Read the model definition and answer for the solid it produces. Units are mm, in the model's axes. A direction names the side the tool comes from. Coordinates: 2 decimals unless noted, no trailing zeros. Order: outer loops, then holes, each group sorted by start corner. A loop starts at its lowest first (then second) coordinate and runs counter-clockwise, first axis right, second up.
```python
from build123d import *

# Parameters (mm, degrees)
F1_W     = 21
F1_H     = 35
F2_DEPTH = 23
F3_W     = 19
F3_H     = 33
F4_DEPTH = 22
F5_W     = 7
F5_H     = 14.7
F6_DEPTH = 25
F8_D     = 4
F8_DEPTH = 6
F8_TIP   = 1.2017212381


with BuildPart() as f2:
    # F1 (on Front) → F2 (new body)
    with BuildSketch(Plane.XZ):
        Rectangle(F1_W, F1_H)
    extrude(amount=-F2_DEPTH)

    # F3 (on face) → F4 (cut)
    with BuildSketch(Plane(origin=(0, 23, 0), x_dir=(-1, 0, 0), z_dir=(0, 1, 0))):
        Rectangle(F3_W, F3_H)
    extrude(amount=-F4_DEPTH, mode=Mode.SUBTRACT)

    # F5 (on Front) → F6 (cut)
    with BuildSketch(Plane.XZ):
        Rectangle(F5_W, F5_H)
    extrude(amount=-F6_DEPTH, mode=Mode.SUBTRACT)

    # F8
    with Locations(Plane.XZ):
        with Locations((0, 14.35), (-6, 0), (6, 0), (0, -14.35)):
            Hole(F8_D / 2, depth=F8_DEPTH)
            with Locations((0, 0, -(F8_DEPTH + F8_TIP / 2))):  # 118° drill point
                Cone(0, F8_D / 2, F8_TIP, mode=Mode.SUBTRACT)


solid = f2.part
```
1) Flat-ended cylindrical pins translate along their axes: pin 1 Ø1.5 at (x, z) = (-1, -9.5) entering from +Y; pin 2 Ø4.5 at (x, z) = (0, 14.35) entering from +Y; pin 3 Ø3.5 at (x, z) = (-6, 0) entering from -Y. Find the tip coordinate at first contact, or state that the pin passes through.
A:
pin 1: stops at y = 1
pin 2: stops at y = 23
pin 3: passes through
2) A cutting plane is placed at D-D, the plane z = 14.35. Determine the outline of the cut face in (x, y).
A:
outline: (-10.5, 0) - (-2, 0) - (-2, 1) - (-9.5, 1) - (-9.5, 23) - (-10.5, 23) - close; (2, 0) - (10.5, 0) - (10.5, 23) - (9.5, 23) - (9.5, 1) - (2, 1) - close
3) A cutting plane is placed at B-B, the plane x = 6. Determine the outline of the cut face in (y, z), and give its area (3 significant figures).
A:
outline: (0, -17.5) - (23, -17.5) - (23, -16.5) - (1, -16.5) - (1, -2) - (0, -2) - close; (0, 2) - (1, 2) - (1, 16.5) - (23, 16.5) - (23, 17.5) - (0, 17.5) - close
area: 75.0 mm2
4) A cutting plane is placed at C-C, the plane y = 21.75. Determine the outline of the cut face in (x, z), and give its area (3 significant figures).
A:
outline: (-10.5, -17.5) - (10.5, -17.5) - (10.5, 17.5) - (-10.5, 17.5) - close; hole (-9.5, -16.5) - (9.5, -16.5) - (9.5, 16.5) - (-9.5, 16.5) - close
area: 108 mm2
5) Straight lines are drawn through the part: line 1 (Z direction, x = 6, y = 0.6); line 2 (Z direction, x = -4.25, y = 17.5); line 3 (Z direction, x = 0, y = 0.7). For each, find the intervals that lie inside material, in ascending order.
A:
line 1: z = -17.5 to -2, 2 to 17.5
line 2: z = -17.5 to -16.5, 16.5 to 17.5
line 3: z = -17.5 to -16.35, -12.35 to -7.35, 7.35 to 12.35, 16.35 to 17.5
6) Which of the six approach directions +Z, -Z, +X, -X, +Y, -Y give full straight-line access (tool end or side, diameter ignored) to faces 1 (the flat face through (0, 12, 16.5)), 2 (the flat face through (3.5, 0.5, -0.1)), 3 (the flat face through (10.5, 11, 0))?
A:
face 1: +Y
face 2: +Y, -Y
face 3: +Z, -Z, +X, +Y, -Y
7) Determine the mould class of faces 4 (the flat face through (-10.5, 11, 0)), 5 (the cylindrical face through (-4.4, 0.5, -1.2)), 6 (the flat face through (0, 11, 17.5)) for opening direction X: pulls with the +X half, pulls with the -X half, needs draft (parallel to the pull), parting line crosses it, or undercut.
A:
face 4: pulls with the -X half
face 5: undercut
face 6: needs draft
8) A cutting plane is placed at A-A, the plane z = 0. Determine the outline of the cut face in (x, y), and give its area (3 significant figures).
A:
outline: (-10.5, 0) - (-8, 0) - (-8, 1) - (-9.5, 1) - (-9.5, 23) - (-10.5, 23) - close; (-4, 0) - (-3.5, 0) - (-3.5, 1) - (-4, 1) - close; (3.5, 0) - (4, 0) - (4, 1) - (3.5, 1) - close; (8, 0) - (10.5, 0) - (10.5, 23) - (9.5, 23) - (9.5, 1) - (8, 1) - close
area: 50.0 mm2
